Here's how the part is built. I have some questions about the finished solid (model axes, mm). Face numbers are marked on the shaded views. A direction names the side the tool comes from. Coordinates: 2 decimals unless noted, no trailing zeros. Write each loop counter-clockwise with the first axis right and the second up, starting at its lowest first coordinate (ties: lowest second). Pieces come first, ordered by that corner, then holes.
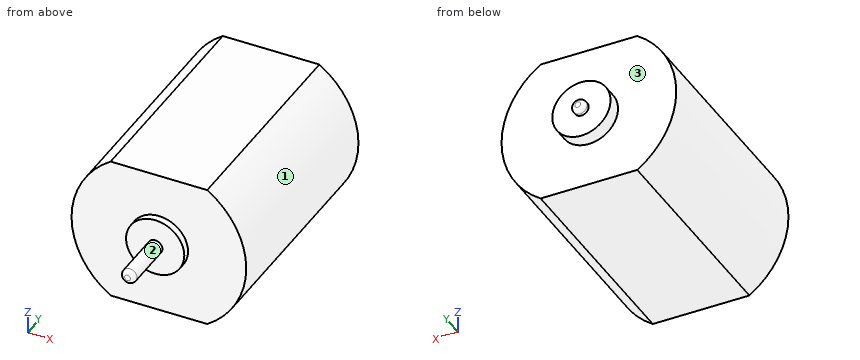
```python
from build123d import *

# Parameters (mm, degrees)
F0_R          = 0.5
F0_R_2        = 2
F1_DEPTH      = 15
F2_DEPTH      = 0.5
F2_DEPTH_BACK = 16
F3_DEPTH      = 4.2
F3_DEPTH_BACK = 16.5
F4_R          = 0.3


with BuildPart() as f1:
    # F0 (on Front) → F1 (new body)
    with BuildSketch(Plane.XZ):
        Circle(F0_R)
        Circle(F0_R_2)
        Circle(F0_R, mode=Mode.SUBTRACT)
        with BuildLine():
            Line((-3.316625, -5), (3.316625, -5))
            ThreePointArc((3.316625, -5), (6, 0), (3.316625, 5))
            Line((3.316625, 5), (-3.316625, 5))
            ThreePointArc((-3.316625, 5), (-6, 0), (-3.316625, -5))
        make_face()
        Circle(F0_R_2, mode=Mode.SUBTRACT)
    extrude(amount=-F1_DEPTH)

    # F0 (on Front) → F2 (join, two sides)
    with BuildSketch(Plane.XZ) as f2_sk:
        Circle(F0_R)
        Circle(F0_R_2)
        Circle(F0_R, mode=Mode.SUBTRACT)
    extrude(amount=F2_DEPTH)
    extrude(f2_sk.sketch, amount=-F2_DEPTH_BACK)

    # F0 (on Front) → F3 (join, two sides)
    with BuildSketch(Plane.XZ) as f3_sk:
        Circle(F0_R)
    extrude(amount=F3_DEPTH)
    extrude(f3_sk.sketch, amount=-F3_DEPTH_BACK)

    # F4
    f4_edges = [f1.edges().sort_by_distance(p)[0] for p in [
        (-0.5, -4.2, 0),
        (-0.5, 16.5, 0),
    ]]
    fillet(f4_edges, radius=F4_R)


solid = f1.part
```
1) Imagine slicing it at A-A on x = -1.25. Please give me the cut outline in (y, z), then the cut area to 3 significant figures.
Values follow:
outline: (-0.5, -1.56) - (0, -1.56) - (0, -5) - (15, -5) - (15, -1.56) - (16, -1.56) - (16, 1.56) - (15, 1.56) - (15, 5) - (0, 5) - (0, 1.56) - (-0.5, 1.56) - close
area: 155 mm2
2) Imagine slicing it at B-B on z = -1.5. Please give me the cut outline in (x, y), then the cut area to 3 significant figures.
Values follow:
outline: (-5.81, 0) - (-1.32, 0) - (-1.32, -0.5) - (1.32, -0.5) - (1.32, 0) - (5.81, 0) - (5.81, 15) - (1.32, 15) - (1.32, 16) - (-1.32, 16) - (-1.32, 15) - (-5.81, 15) - close
area: 178 mm2
3) Imagine slicing it at D-D on z = -3.75. Please give me the cut outline in (x, y), then the cut area to 3 significant figures.
Values follow:
outline: (-4.68, 0) - (4.68, 0) - (4.68, 15) - (-4.68, 15) - close
area: 141 mm2
4) I need wall thicknesses on probe 1 along Y at (x, z) = (2.5, 2.25); probe 2 along Y at (x, z) = (1.5, -1.25); probe 3 along X at (y, z) = (14.25, 2). Which ranges of each line are inside material? Lowest first, please.
Values follow:
probe 1: y = 0 to 15
probe 2: y = -0.5 to 16
probe 3: x = -5.66 to 5.66
5) Will these pins go through, and if not, where does the flat tip stop? pin 1 (1.5 mm diameter, centred on y = 1, z = 2.5, fed in from +X); pin 2 (1 mm diameter, centred on x = 2, z = 1, fed in from -Y); pin 3 (1 mm diameter, centred on x = 4, z = 1, fed in from -Y).
Values follow:
pin 1: stops at x = 5.74
pin 2: stops at y = -0.5
pin 3: stops at y = 0
6) Imagine slicing it at C-C on y = 12.5. Please give me the cut outline in (x, z).
Values follow:
outline: (-3.32, -5) - (3.32, -5) arc R6 ccw to (3.32, 5) - (-3.32, 5) arc R6 ccw to start
7) On a 3-axis mill with a long thin cutter (end or side, diameter ignored), from which of +Z, -Z, +X, -X, +Y, -Y can I reach the whole of each face in a straight line? I mean the marked faces 1, 2 and 3. Say none if no direction works.
Values follow:
face 1: +X, +Y, -Y
face 2: -Y
face 3: +Y
